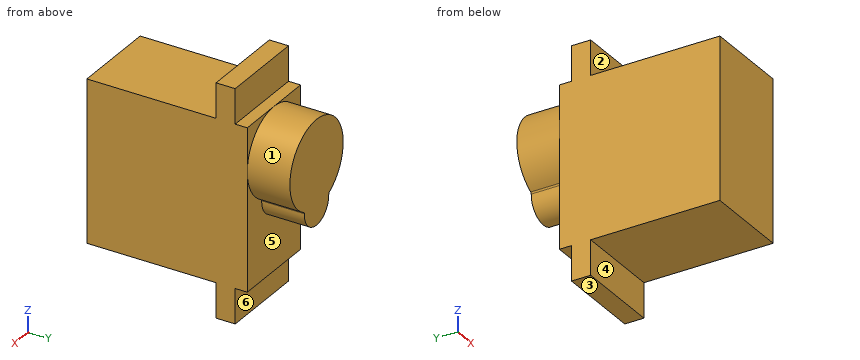
Autodesk Inventor part; units mm, degrees
ref_plane "YZ Plane" through (0, 0, 0) normal (1, 0, 0) x (0, 1, 0)
ref_plane "XZ Plane" through (0, 0, 0) normal (0, 1, 0) x (-1, 0, 0)
ref_plane "XY Plane" through (0, 0, 0) normal (0, 0, 1) x (1, 0, 0)
sketch "Sketch1" plane through (0, 0, 0) normal (0, 1, 0) x (-1, 0, 0)
  line L0 (0, 0) -> (12.2, 0)
  line L1 (12.2, 0) -> (12.2, -22.7)
  line L2 (12.2, -22.7) -> (0, -22.7)
  line L3 (0, -22.7) -> (0, 0)
  dimension "d0" = 12.2
  dimension "d1" = 22.7
extrude "Extrusion1" add sketch "Sketch1" along normal blind 18.2
sketch "Sketch2" plane through (0, 18.2, 0) normal (0, 1, 0) x (1, 0, 0)
  line L0 (-12.2, -4.9) -> (0, -4.9)
  line L1 (0, -4.9) -> (0, 27.6)
  line L2 (0, 27.6) -> (-12.2, 27.6)
  line L3 (-12.2, 27.6) -> (-12.2, -4.9)
  line L4 (-12.2, -4.9) -> (0, 27.6) construction
  line L5 (0, -4.9) -> (-12.2, 27.6) construction
  line L6 (-12.2, 0) -> (0, 0)
  line L7 (-12.2, 22.7) -> (-12.2, 0)
  point P0 (-6.1, 11.35)
  dimension "d4" = 32.5
  dimension "d5" = 12.2
  dimension "d6" = 11.35
  dimension "d7" = 6.1
extrude "Extrusion2" add sketch "Sketch2" along normal blind 2.7
sketch "Sketch3" plane through (0, 20.9, 0) normal (0, 1, 0) x (1, 0, 0)
  line L0 (0, 22.7) -> (-12.2, 22.7)
  line L1 (0, 0) -> (-12.2, 0)
  line L2 (-12.2, 0) -> (-12.2, 22.7)
  line L3 (-12.2, 22.7) -> (0, 22.7)
  line L4 (0, 22.7) -> (0, 0)
extrude "Extrusion3" add sketch "Sketch3" along normal blind 1.7
sketch "Sketch5" plane through (0, 22.6, 0) normal (0, 1, 0) x (1, 0, 0)
  circle A0 centre (-6.1, 6.1) radius 6.1
  line L0 (-12.2, 22.7) -> (-12.2, 0)
  line L1 (0, 0) -> (0, 22.7)
  line L2 (-12.2, 0) -> (0, 0)
  circle A1 centre (-6.1, 11.8) radius 2.8
  point P0 (-8.8866, 11.5263)
  point P1 (-3.3134, 11.5263)
  dimension "d12" = 6.1
  dimension "d13" = 5.6
  dimension "d14" = 14.6
extrude "Extrusion4" add sketch "Sketch5" along normal blind 6 contours A0 A1 | A1 A0 | A0 A1
fillet "Fillet1" radius 0.25 2 edges at (-8.8866, 25.6, -11.5263) (-3.3134, 25.6, -11.5263)
properties part number "Servo"
Design review of the part built by this model. Coordinates are the model's own, in mm. Face numbers are marked on the shaded views. A direction names the side the tool comes from. Give positions to 0.01 mm unless a question says otherwise; leave off trailing zeros. Loops run counter-clockwise (first coordinate to the right, second up) from the corner with the lowest first, then second, coordinate; pieces in that order, holes last. Notation, with made-up numbers: M 43,-25 L 85,-25 A7 cw 85,-17 Z; hole C 16.5,63.25 d9. An arc over 180 degrees is marked long. Answer as a JSON object with one key per item and string values.
Item 1: Machinability: for the marked faces 4, 5 and 6, which of the approach directions +Z, -Z, +X, -X, +Y, -Y give a long, thin tool a straight path to every point of the face, cutting with its end or side? Answer none if there is none.
Output values:
{"face 4": "-Z, +X, -X, -Y", "face 5": "-Z, +Y", "face 6": "-Z, +X, -X, +Y"}
Item 2: We need section B-B (z = -20). State the section outline as (x, y) points.
Output values:
{"outline": "M -12.2,0 L 0,0 L 0,22.6 L -12.2,22.6 Z"}
Item 3: We need section C-C (y = 8). State the section outline as (x, z) points, and give its area (3 significant figures).
Output values:
{"outline": "M -12.2,-22.7 L 0,-22.7 L 0,0 L -12.2,0 Z", "area": "277 mm2"}
Item 4: Mouldability with a two-part tool opening along Z and no side actions: class the marked faces 1, 2 and 3 as pulls with the +Z half, pulls with the -Z half, needs draft (parallel to the pull), parting line crosses it, or undercut.
Output values:
{"face 1": "parting line crosses it", "face 2": "needs draft", "face 3": "pulls with the -Z half"}
Item 5: Wall thickness on line 1 along Z through (x, y) = (-6, 10.5); line 2 along Y through (x, z) = (-7, 3.5); line 3 along Y through (x, z) = (-3.75, -19.5): over which ranges is each line inside the solid? List them lowest first.
Output values:
{"line 1": "z = -22.7 to 0", "line 2": "y = 18.2 to 20.9", "line 3": "y = 0 to 22.6"}
Item 6: For P1, Ø0.9, axis at x = -4.5, y = 22, coming from the -Z side; P2, Ø1.5, axis at x = -7.5, y = 11, coming from the +Z side; P3, Ø2.5, axis at x = -6, z = -24.5, coming from the +Y side, all flat-tipped, find the tip position at first contact; note any pin that passes through.
Output values:
{"P1": "stops at z = -22.7", "P2": "stops at z = 0", "P3": "stops at y = 20.9"}
Item 7: We need section A-A (x = -9.75). State the section outline as (y, z) points, and give its area (3 significant figures).
Output values:
{"outline": "M 0,-22.7 L 18.2,-22.7 L 18.2,-27.6 L 20.9,-27.6 L 20.9,-22.7 L 22.6,-22.7 L 22.6,-10.99 L 28.6,-10.99 L 28.6,-1.21 L 22.6,-1.21 L 22.6,0 L 20.9,0 L 20.9,4.9 L 18.2,4.9 L 18.2,0 L 0,0 Z", "area": "598 mm2"}
Item 8: We need section D-D (x = -4.5). State the section outline as (y, z) points, and give its area (3 significant figures).
Output values:
{"outline": "M 0,-22.7 L 18.2,-22.7 L 18.2,-27.6 L 20.9,-27.6 L 20.9,-22.7 L 22.6,-22.7 L 22.6,-14.1 L 28.6,-14.1 L 28.6,-0.21 L 22.6,-0.21 L 22.6,0 L 20.9,0 L 20.9,4.9 L 18.2,4.9 L 18.2,0 L 0,0 Z", "area": "623 mm2"}
